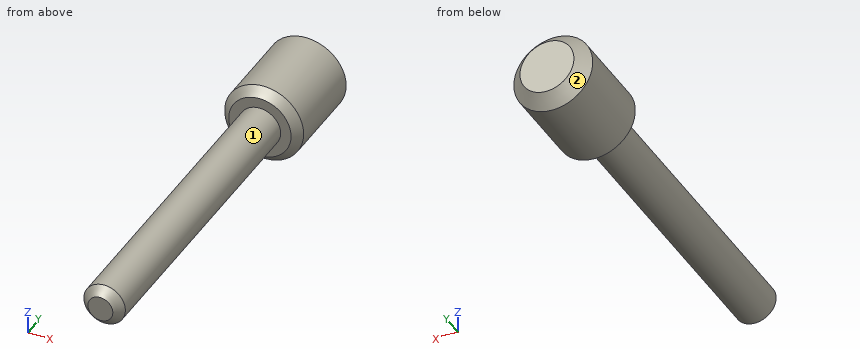
Autodesk Inventor part; units mm, degrees
ref_plane "YZ Plane" through (0, 0, 0) normal (1, 0, 0) x (0, 1, 0)
ref_plane "XZ Plane" through (0, 0, 0) normal (0, 1, 0) x (-1, 0, 0)
ref_plane "XY Plane" through (0, 0, 0) normal (0, 0, 1) x (1, 0, 0)
sketch "Sketch2" plane through (0, 0, 0) normal (0, 1, 0) x (-1, 0, 0)
  circle A0 centre (0, 0) radius 5
  dimension "d7" = 10
extrude "Extrusion1" add sketch "Sketch2" along normal blind 75
sketch "Sketch3" plane through (0, 75, 0) normal (0, 1, 0) x (1, 0, 0)
  circle A0 centre (0, 0) radius 9.5
  dimension "d10" = 19
extrude "Extrusion2" add sketch "Sketch3" along normal blind 25
sketch "Sketch4" plane through (0, 0, 0) normal (1, 0, 0) x (0, 1, 0)
  point P0 (0, 0)
chamfer "Chamfer1" distance 2 angle 45 1 edges at (5, 0, 0)
chamfer "Chamfer2" distance 3 angle 45 1 edges at (-9.5, 100, 0)
chamfer "Chamfer3" distance 2 angle 45 1 edges at (-9.5, 75, 0)
equation "\"BendRadius\" = Thickness"
equation "\"BendReliefWidth\" = Thickness"
equation "\"BendReliefDepth\" = 0.5 * Thickness"
equation "\"CornerReliefSize\" = 4 * Thickness"
equation "\"MinimumRemnant\" = 2 * Thickness"
equation "\"TransitionRadius\" = BendRadius"
equation "\"JacobiRadiusSize\" = BendRadius"
equation "\"GapSize\" = Thickness"
properties part number "BOLT" material "Stainless Steel"
The model under review builds one solid part; all positions refer to its coordinate system, in mm. Face numbers are marked on the shaded views. A direction names the side the tool comes from. Give positions to 0.01 mm unless a question says otherwise; leave off trailing zeros. Order: outer loops, then holes, each group sorted by start corner. A loop starts at its lowest first (then second) coordinate and runs counter-clockwise, first axis right, second up. Notation, with made-up numbers: M -13,-2 L -4,-2 A26 ccw -4,23 Z; hole C 81,-9.5 d10. An arc over 180 degrees is marked long. Answer in a Markdown table with one row per item. Add a question column.
1. Add section A-A on z = 0. State the section outline as (x, y) points, plus the area to 3 significant figures.
2. To check wall thickness, follow line 1 along Y through (x, z) = (4.5, -3); line 2 along Z through (x, y) = (4, 59.5); line 3 along Y through (x, z) = (6.75, -2.5). State the ranges of each line that lie inside material, in increasing order.
3. Add section C-C on y = 59. State the section outline as (x, z) points.
4. For pin 1 Ø1.5 at (x, y) = (4, 48) entering from -Z; pin 2 Ø1.5 at (y, z) = (69.5, 0.5) entering from -X; pin 3 Ø1 at (x, y) = (-2, 75) entering from +Z; pin 4 Ø3 at (x, y) = (-0.5, 84) entering from +Z, all flat-tipped, find the tip position at first contact; note any pin that passes through.
5. Machinability: for the marked faces 1 and 2, which of the approach directions +Z, -Z, +X, -X, +Y, -Y give a long, thin tool a straight path to every point of the face, cutting with its end or side? Answer none if there is none.
6. Add section B-B on x = 0. State the section outline as (y, z) points.
The answers:
| question | item | result |
|---|---|---|
| 1 | outline | M -9.5,77 L -7.5,75 L -5,75 L -5,2 L -3,0 L 3,0 L 5,2 L 5,75 L 7.5,75 L 9.5,77 L 9.5,97 L 6.5,100 L -6.5,100 L -9.5,97 Z |
| 1 | area | 1,210 mm2 |
| 2 | line 1 | 75 to 100 |
| 2 | line 2 | -3 to 3 |
| 2 | line 3 | 75 to 99.3 |
| 3 | outline | C 0,0 d10 |
| 4 | pin 1 | z = -3.8 |
| 4 | pin 2 | x = -5 |
| 4 | pin 3 | z = 7.76 |
| 4 | pin 4 | z = 9.5 |
| 5 | face 1 | -Y |
| 5 | face 2 | +Y |
| 6 | outline | M 0,-3 L 2,-5 L 75,-5 L 75,-7.5 L 77,-9.5 L 97,-9.5 L 100,-6.5 L 100,6.5 L 97,9.5 L 77,9.5 L 75,7.5 L 75,5 L 2,5 L 0,3 Z |
